Source: CAD feature listing. Evaluate the final solid. Frame: model axes, mm. Round coordinates to 2 decimals unless told otherwise and drop trailing zeros. Loops run counter-clockwise (first coordinate to the right, second up) from the corner with the lowest first, then second, coordinate; pieces in that order, holes last.
(1) Section D-D, the plane z = 63. Return the cut outline in (x, y), plus the area to 3 significant figures.
(2) First-contact query: pin 1 Ø2 at (y, z) = (-14.5, -68.5) entering from -X; pin 2 Ø12 at (x, y) = (-46.5, -80.5) entering from +Z; pin 3 Ø1.5 at (x, y) = (-11, -77) entering from +Z. Flat tips, straight axial feed; report the tip coordinate or a pass-through.
(3) Section A-A, the plane x = 0. Return the cut outline in (y, z).
(4) Section B-B, the plane z = 0. Return the cut outline in (x, y).
(5) Material intervals for probe 1 along Z at (x, y) = (-40, -38.5); probe 2 along Z at (x, y) = (30.5, -6.5); probe 3 along X at (y, z) = (-63.5, -39), sorted ascending.
(6) Section C-C, the plane y = -82.5. Return the cut outline in (x, z).
```python
from build123d import *

# Parameters (mm, degrees)
SKETCH_2_R          = 100
CUT_EXTRUDE_1_DEPTH = 101
SKETCH_3_R          = 2.5
CUT_EXTRUDE_2_DEPTH = 101


with BuildPart() as part:
    # 草图1 → 旋转1 (revolve)
    with BuildSketch(Plane.XY):
        with BuildLine():
            Line((-100, 0), (-98, 0))
            ThreePointArc((-98, 0), (0, -98), (98, 0))
            Line((98, 0), (100, 0))
            ThreePointArc((100, 0), (0, -100), (-100, 0))
        make_face()
    revolve(axis=Axis((-100, 0, 0), (1, 0, 0)))

    # 草图2 → 切除-拉伸1 (cut, through all)
    with BuildSketch(Plane(origin=(0, 0, 0), x_dir=(1, 0, 0), z_dir=(0, 1, 0))):
        Circle(SKETCH_2_R)
    extrude(amount=CUT_EXTRUDE_1_DEPTH, mode=Mode.SUBTRACT)

    # 草图3 → 切除-拉伸2 (cut, through all)
    with BuildSketch(Plane(origin=(0, 0, 0), x_dir=(1, 0, 0), z_dir=(0, 1, 0))):
        Circle(SKETCH_3_R)
    extrude(amount=-CUT_EXTRUDE_2_DEPTH, mode=Mode.SUBTRACT)


solid = part.part
```
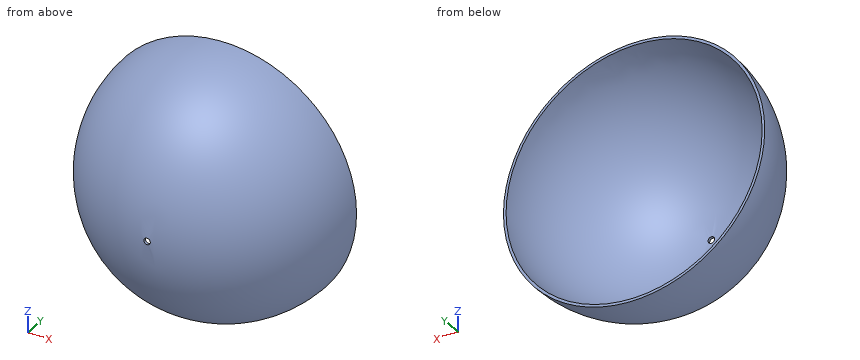
Output values:
1. outline: (-77.66, 0) arc R77.66 ccw to (77.66, 0) - (75.07, 0) arc R75.07 cw to (-75.07, 0) - close
1. area: 622 mm2
2. pin 1: stops at x = -72.36
2. pin 2: stops at z = 49.37
2. pin 3: stops at z = 63.77
3. outline: (-99.97, -2.5) arc R100 ccw to (0, -100) - (0, -98) arc R98 cw to (-97.97, -2.5) - close; (-99.97, 2.5) - (-97.97, 2.5) arc R98 cw to (0, 98) - (0, 100) arc R100 ccw to start
4. outline: (-100, 0) arc R100 ccw to (-2.5, -99.97) - (-2.5, -97.97) arc R98 cw to (-98, 0) - close; (2.5, -99.97) arc R100 ccw to (100, 0) - (98, 0) arc R98 cw to (2.5, -97.97) - close
5. probe 1: z = -83.17 to -80.76, 80.76 to 83.17
5. probe 2: z = -95.01 to -92.91, 92.91 to 95.01
5. probe 3: x = -66.68 to -63.65, 63.65 to 66.68
6. outline: circle Ø113.03 at (0, 0); hole circle Ø105.79 at (0, 0)
